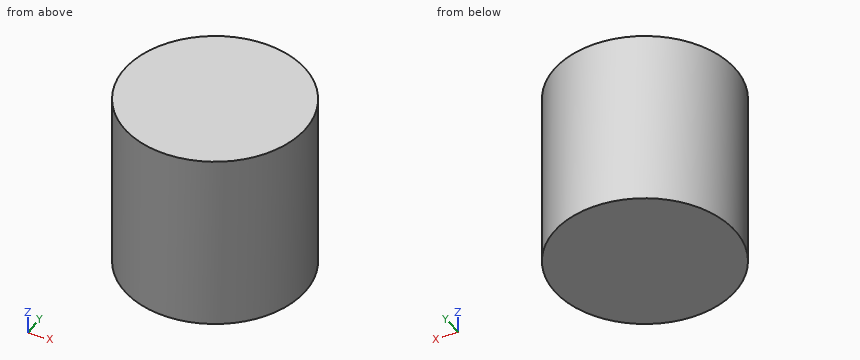
from build123d import *

# Parameters (mm, degrees)
F0_W     = 69.465278
F0_H     = 106.150199
F1_DEPTH = 25.4
F2_R     = 5.08
F3_R     = 12.783767
F4_DEPTH = 25.4


with BuildPart() as f1:
    # F0 (on Top) → F1 (new body)
    with BuildSketch(Plane.XY):
        with Locations((-1.492229, 2.367309)):
            Rectangle(F0_W, F0_H)
    extrude(amount=F1_DEPTH)

    # F2
    f2_edges = [f1.edges().sort_by_distance(p)[0] for p in [
        (33.24041, 2.367308, 25.4),
        (-1.492229, -50.707791, 25.4),
        (-36.224868, 2.367308, 25.4),
        (-1.492229, 55.442408, 25.4),
        (33.24041, -50.707791, 12.7),
        (33.24041, 55.442408, 12.7),
        (-36.224868, -50.707791, 12.7),
        (-36.224868, 55.442408, 12.7),
    ]]
    fillet(f2_edges, radius=F2_R)

    # F3 (on face) → F4 (intersect)
    with BuildSketch(Plane.XY.offset(25.4)):
        with Locations((-4.704368, -7.827024)):
            Circle(F3_R)
    extrude(amount=-F4_DEPTH, mode=Mode.INTERSECT)


solid = f1.part
Input: part model. Units: mm. Frame: model coordinates. Give positions to 0.01 mm unless a question says otherwise; leave off trailing zeros. Order: outer loops, then holes, each group sorted by start corner. A loop starts at its lowest first (then second) coordinate and runs counter-clockwise, first axis right, second up. Notation, with made-up numbers: M -25.5,42.25 L -11.5,42.25 A11 ccw -11.5,61.25 Z; hole C 33,37.5 d7. An arc over 180 degrees is marked long. Answer as a JSON object with one key per item and string values.
1. First-contact query: P1, Ø8, axis at x = 2.5, z = 11.5, coming from the -Y side; P2, Ø1, axis at y = -5.5, z = 8.5, coming from the -X side; P3, Ø4, axis at x = -10, z = 7, coming from the +Y side. Flat tips, straight axial feed; report the tip coordinate or a pass-through.
Result sheet:
{"P1": "y = -20.2", "P2": "x = -17.36", "P3": "y = 4.52"}
2. Cut plane B-B, the plane y = -4.75. Output: boundary loops of the cut face in (x, z).
Result sheet:
{"outline": "M -17.11,0 L 7.7,0 L 7.7,25.4 L -17.11,25.4 Z"}
3. Cut plane C-C, the plane z = 5.5. Output: boundary loops of the cut face in (x, y), and give its area (3 significant figures).
Result sheet:
{"outline": "C -4.7,-7.83 d25.57", "area": "513 mm²"}
4. Ray query, line 1 (X direction, y = -7.75, z = 4.25); line 2 (X direction, y = -15, z = 23.25); line 3 (Y direction, x = -1.25, z = 23.5). Return the intervals inside material, ascending. Write a range as [from, to].
Result sheet:
{"line 1": "[-17.49, 8.08]", "line 2": "[-15.29, 5.88]", "line 3": "[-20.14, 4.48]"}
5. Cut plane A-A, the plane x = -8.5. Output: boundary loops of the cut face in (y, z).
Result sheet:
{"outline": "M -20.03,0 L 4.38,0 L 4.38,25.4 L -20.03,25.4 Z"}
